Autodesk Inventor part; units mm, degrees
ref_plane "YZ Plane" through (0, 0, 0) normal (1, 0, 0) x (0, 1, 0)
ref_plane "XZ Plane" through (0, 0, 0) normal (0, 1, 0) x (-1, 0, 0)
ref_plane "XY Plane" through (0, 0, 0) normal (0, 0, 1) x (1, 0, 0)
sketch "Sketch1" plane through (0, 0, 0) normal (1, 0, 0) x (0, 1, 0)
  line L0 (0, 0) -> (1.65, 0) construction
  line L1 (1.65, 0) -> (3, 0) construction
  line L2 (4.95, 0) -> (4.95, -1.5)
  line L3 (4.95, -1.5) -> (3.95, -1.5)
  line L4 (3.95, -1.5) -> (3.95, -16)
  line L5 (3.95, -16) -> (1.6, -16)
  line L6 (1.6, -16) -> (1.6, -3)
  line L7 (0, 0) -> (0, -13.7466) construction
  line L8 (3, 0) -> (3, -3)
  line L9 (3, -3) -> (1.6, -3)
  line L10 (3, 0) -> (4.95, 0)
  dimension "d0" = 1.6
  dimension "d1" = 3.95
  dimension "d2" = 1
  dimension "d3" = 1.5
  dimension "d4" = 14.5
  dimension "d6" = 3
  dimension "d7" = 3
revolve "Revolution1" add sketch "Sketch1" angle 360 about axis through (0, 0, 0) along (0, 0, -1)
fillet "Fillet1" radius 0.5 2 edges at (0, -1.6, -16) (0, -3.95, -16)
properties part number "HD_BearingShaft2"
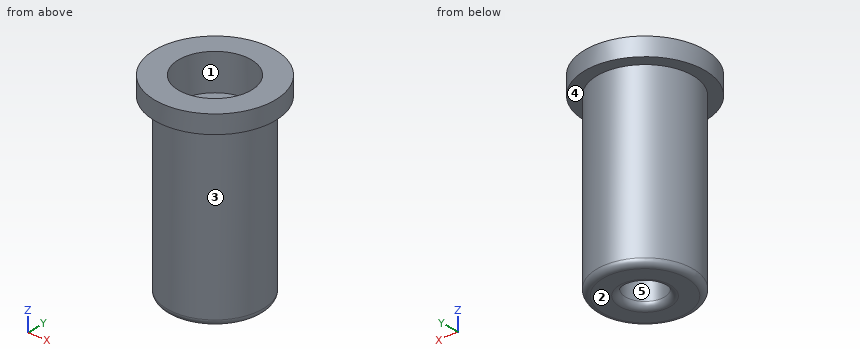
The model under review builds one solid part; all positions refer to its coordinate system, in mm. Face numbers are marked on the shaded views. A direction names the side the tool comes from. Round coordinates to 2 decimals unless told otherwise and drop trailing zeros. Write each loop counter-clockwise with the first axis right and the second up, starting at its lowest first coordinate (ties: lowest second). Pieces come first, ordered by that corner, then holes. Notation, with made-up numbers: (-17, 81) - (39, 81) arc R32 cw to (39, 117) - close; hole circle Ø2 at (-34.5, 12). An arc over 180 degrees is marked (long way). Answer as CSV lines item,"result". Start each with the question number.
(1) For the marked faces 4 and 5, list the 3-axis set-ups (+Z, -Z, +X, -X, +Y, -Y) from which the entire face can be reached by the end or side of a thin tool; tool diameter is ignored.
(2) We need section D-D on y = 4.5. State the section outline as (x, z) points.
(3) Draft analysis for pull direction Y (two halves, no side actions). For the marked faces 1, 2 and 3, state which applies: pulls with the +Y half, pulls with the -Y half, needs draft (parallel to the pull), parting line crosses it, or undercut.
(4) We need section C-C on z = -4. State the section outline as (x, y) points, plus the area to 3 significant figures.
(5) To check wall thickness, follow line 1 (X direction, y = 0, z = -8); line 2 (X direction, y = 0, z = -1.05); line 3 (Z direction, x = -2.5, y = 1). State the ranges of each line that lie inside material, in increasing order.
(6) For pin 1 Ø3.5 at (x, y) = (0, 0) entering from -Z; pin 2 Ø1.5 at (x, z) = (-3, -10) entering from -Y; pin 3 Ø4 at (x, z) = (2, -13.5) entering from +Y, all flat-tipped, find the tip position at first contact; note any pin that passes through.
(7) We need section A-A on y = 0. State the section outline as (x, z) points, plus the area to 3 significant figures.
Worked answers:
1,face 4,"-Z"
1,face 5,"+Z, -Z"
2,outline,"(-2.06, -1.5) - (2.06, -1.5) - (2.06, 0) - (-2.06, 0) - close"
3,face 1,"undercut"
3,face 2,"needs draft"
3,face 3,"parting line crosses it"
4,outline,"circle Ø7.9 at (0, 0); hole circle Ø3.2 at (0, 0)"
4,area,"41.0 mm²"
5,line 1,"-3.95 to -1.6, 1.6 to 3.95"
5,line 2,"-4.95 to -3, 3 to 4.95"
5,line 3,"-16 to -3"
6,pin 1,"z = -15.86"
6,pin 2,"y = -3.25"
6,pin 3,"y = 3.95"
7,outline,"(-4.95, -1.5) - (-3.95, -1.5) - (-3.95, -15.5) arc R0.5 ccw to (-3.45, -16) - (-2.1, -16) arc R0.5 ccw to (-1.6, -15.5) - (-1.6, -3) - (-3, -3) - (-3, 0) - (-4.95, 0) - close; (1.6, -15.5) arc R0.5 ccw to (2.1, -16) - (3.45, -16) arc R0.5 ccw to (3.95, -15.5) - (3.95, -1.5) - (4.95, -1.5) - (4.95, 0) - (3, 0) - (3, -3) - (1.6, -3) - close"
7,area,"69.6 mm²"
